Read the model definition and answer for the solid it produces. Units are mm, in the model's axes. Round coordinates to 2 decimals unless told otherwise and drop trailing zeros. Order: outer loops, then holes, each group sorted by start corner. A loop starts at its lowest first (then second) coordinate and runs counter-clockwise, first axis right, second up. Notation, with made-up numbers: (84, 67.5) - (104, 67.5) arc R28 cw to (104, 93.5) - close; hole circle Ø10 at (88, -36.75). An arc over 180 degrees is marked (long way). Put each result on its own line as item: value. Start each with the question number.
Q1. Section B-B on z = 0.85 is taken. Give the vertices of the cut face in (x, y).
Q2. Section C-C on x = 5.25 is taken. Give the vertices of the cut face in (y, z).
Q3. Find the intervals of material crossed by line 1 along Y through (x, z) = (5, 0.6); line 2 along Y through (x, z) = (3.75, 1.45); line 3 along X through (y, z) = (86, 1.9), in increasing order. Write a range as from..to.
Q4. This flat-tipped pin is pushed along its axis until it touches: pin 1 Ø4 at (x, y) = (8.5, 48.5) entering from -Z. Where does it stop, or does it pass through?
Q5. Section A-A on y = 85.5 is taken. Give the vertices of the cut face in (x, z), then the cut area to 4 significant figures.
from build123d import *

# Parameters (mm, degrees)
SKETCH1_W           = 10
SKETCH1_H           = 100
BOSS_EXTRUDE1_DEPTH = 2.5
SKETCH2_R           = 3
CUT_EXTRUDE1_DEPTH  = 101.529846314
SKETCH5_R           = 3
CUT_EXTRUDE2_DEPTH  = 101.529846314
SKETCH3_R           = 3
CUT_EXTRUDE3_DEPTH  = 10


with BuildPart() as part:
    # Sketch1 → Boss-Extrude1 (new body)
    with BuildSketch(Plane.XY):
        with Locations((5, 50)):
            Rectangle(SKETCH1_W, SKETCH1_H)
    extrude(amount=BOSS_EXTRUDE1_DEPTH)

    # Sketch2 → Cut-Extrude1 (cut, through all)
    with BuildSketch(Plane.XY.offset(2.5)):
        with Locations((5, 4.5)):
            Circle(SKETCH2_R)
    extrude(amount=-CUT_EXTRUDE1_DEPTH, mode=Mode.SUBTRACT)

    # Sketch5 → Cut-Extrude2 (cut, through all)
    with BuildSketch(Plane.XY.offset(2.5)):
        with Locations((5.115048416, 85.5)):
            Circle(SKETCH5_R)
    extrude(amount=-CUT_EXTRUDE2_DEPTH, mode=Mode.SUBTRACT)

    # Sketch3 → Cut-Extrude3 (cut)
    with BuildSketch(Plane.XY.offset(2.5)):
        with Locations((5.115048416, 95.5)):
            Circle(SKETCH3_R)
    extrude(amount=-CUT_EXTRUDE3_DEPTH, mode=Mode.SUBTRACT)


solid = part.part
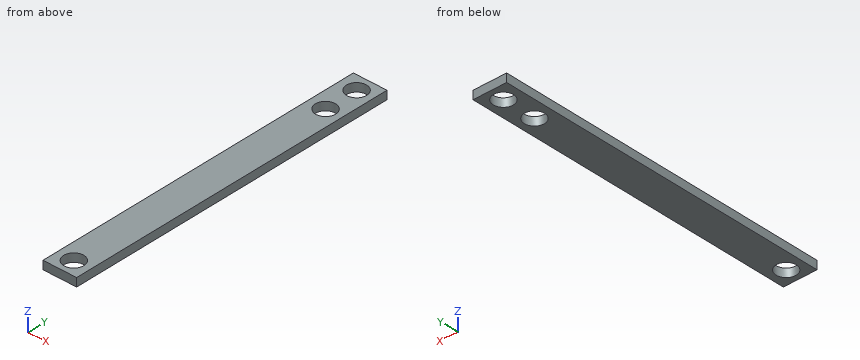
Findings:
1. outline: (0, 0) - (10, 0) - (10, 100) - (0, 100) - close; hole circle Ø6 at (5, 4.5); hole circle Ø6 at (5.12, 85.5); hole circle Ø6 at (5.12, 95.5)
2. outline: (0, 0) - (1.51, 0) - (1.51, 2.5) - (0, 2.5) - close; (7.49, 0) - (82.5, 0) - (82.5, 2.5) - (7.49, 2.5) - close; (88.5, 0) - (92.5, 0) - (92.5, 2.5) - (88.5, 2.5) - close; (98.5, 0) - (100, 0) - (100, 2.5) - (98.5, 2.5) - close
3. line 1: 0..1.5, 7.5..82.5, 88.5..92.5, 98.5..100
3. line 2: 0..1.77, 7.23..82.83, 88.17..92.83, 98.17..100
3. line 3: 0..2.16, 8.07..10
4. pin 1: z = 0
5. outline: (0, 0) - (2.12, 0) - (2.12, 2.5) - (0, 2.5) - close; (8.12, 0) - (10, 0) - (10, 2.5) - (8.12, 2.5) - close
5. area: 10.00 mm2
